Autodesk Inventor part; units mm, degrees
ref_plane "YZ Plane" through (0, 0, 0) normal (1, 0, 0) x (0, 1, 0)
ref_plane "XZ Plane" through (0, 0, 0) normal (0, 1, 0) x (-1, 0, 0)
ref_plane "XY Plane" through (0, 0, 0) normal (0, 0, 1) x (1, 0, 0)
sketch "Sketch1" plane through (0, 0, 0) normal (0, 0, 1) x (1, 0, 0)
  circle A0 centre (10, 20.7) radius 1.6
  line L0 (0, 0) -> (20.0001, 0)
  line L1 (0, 0) -> (0, 7)
  line L2 (20.0001, 0) -> (20.0001, 6.9998)
  line L3 (0, 7) -> (5.4723, 22.0351)
  line L4 (0, 7) -> (16, 7) construction
  line L5 (20.0001, 6.9998) -> (14.5277, 22.0349)
  line L6 (20.0001, 6.9998) -> (36.0001, 6.9998) construction
  arc A1 (14.5277, 22.0349) -> (5.4723, 22.0351) centre (10, 20.3869) ccw
  dimension "d17" = 7
  dimension "d18" = 6.9998
  dimension "d19" = 20.7
  dimension "d23" = 90
  dimension "d24" = 90
  dimension "d25" = 10
  dimension "d26" = 16
  dimension "d27" = 70
  dimension "d28" = 16
  dimension "d29" = 110
  dimension "d30" = 10
sketch "Sketch3" plane through (0, 0, 0) normal (0, 0, 1) x (1, 0, 0)
  point P0 (0, 0)
extrude "Extrusion1" add sketch "Sketch1" along normal blind 4.5
sketch "Sketch4" plane through (0, 0, 4.5) normal (0, 0, 1) x (1, 0, 0)
  line L0 (0, 7) -> (0, 0)
  line L1 (20.0001, 0) -> (20.0001, 6.9998)
  line L2 (0, 0) -> (20.0001, 0)
  line L3 (20.0001, 0) -> (20.0001, 6.9998)
  line L4 (3.884, 22.9404) -> (-0.0481, 7.0119)
  line L5 (20.0001, 6.9998) -> (0, 6.9998)
  line L6 (0, 7) -> (0, 0)
extrude "Extrusion2" add sketch "Sketch4" along normal blind 4.5
sketch "Sketch5" plane through (0, 0, 0) normal (0, -1, 0) x (1, 0, 0)
  circle A0 centre (5, 4) radius 0.5
  circle A1 centre (15, 4) radius 0.5
  line L0 (0, 0) -> (20.0001, 0)
  line L1 (0, 9) -> (20.0001, 9)
  dimension "d13" = 1
  dimension "d14" = 1
  dimension "d33" = 5
  dimension "d34" = 5
extrude "Extrusion3" cut sketch "Sketch5" against normal blind 5.5
properties part number "upper_deck_shaft_mount_for_AD"
Geometry: final body of the model. Coordinates: model frame, mm. A direction names the side the tool comes from. Coordinates: 2 decimals unless noted, no trailing zeros. Order: outer loops, then holes, each group sorted by start corner. A loop starts at its lowest first (then second) coordinate and runs counter-clockwise, first axis right, second up. Notation, with made-up numbers: M -28,41.5 L 21,41.5 A12 ccw 21,58.5 Z; hole C 75.25,75.25 d6. An arc over 180 degrees is marked long. Answer as CSV lines item,"result".
Q1. Section C-C on x = 9.25. Return the cut outline in (y, z), and give its area (3 significant figures).
Answers:
outline,"M 0,0 L 19.29,0 L 19.29,4.5 L 7,4.5 L 7,9 L 0,9 Z; M 22.11,0 L 25.15,0 L 25.15,4.5 L 22.11,4.5 Z"
area,"132 mm^2"
Q2. Section D-D on z = 4. Return the cut outline in (x, y).
Answers:
outline,"M 0,0 L 4.5,0 L 4.5,5.5 L 5.5,5.5 L 5.5,0 L 14.5,0 L 14.5,5.5 L 15.5,5.5 L 15.5,0 L 20,0 L 20,7 L 14.53,22.03 A4.82 ccw 5.47,22.04 L 0,7 Z; hole C 10,20.7 d3.2"
Q3. Line query: probe 1 along Z at (x, y) = (5, 2.45); probe 2 along Y at (x, z) = (10, 2.25); probe 3 along Z at (x, y) = (16, 8.75). Output: solid intervals per line, ascending. Write a range as [from, to].
Answers:
probe 1,"z = [0, 3.5], [4.5, 9]"
probe 2,"y = [0, 19.1], [22.3, 25.21]"
probe 3,"z = [0, 4.5]"
Q4. First-contact query: P1, Ø5, axis at x = 14, z = 7.5, coming from the +Y side; P2, Ø4, axis at y = 17.5, z = 4, coming from the -X side; P3, Ø1.5, axis at x = 7, y = 16.5, coming from the +Z side. Flat tips, straight axial feed; report the tip coordinate or a pass-through.
Answers:
P1,"stops at y = 7"
P2,"stops at x = 3.09"
P3,"stops at z = 4.5"
Q5. Set-up query: faces 5 (the cylindrical face through (8.73, 21.67, 2.22)), 6 (the cylindrical face through (14.935, 2.712, 4.496)), 7 (the flat face through (10, 14, 4.5)). Return all of +Z, -Z, +X, -X, +Y, -Y with unobstructed straight access to the full face (end or side cutting, diameter ignored); none if empty.
Answers:
face 5,"+Z, -Z"
face 6,"-Y"
face 7,"+Z, +X, -X, +Y"
Q6. Section B-B on y = 20.7. Return the cut outline in (x, z).
Answers:
outline,"M 4.99,0 L 8.4,0 L 8.4,4.5 L 4.99,4.5 Z; M 11.6,0 L 15.01,0 L 15.01,4.5 L 11.6,4.5 Z"
Q7. Section A-A on z = 1. Return the cut outline in (x, y).
Answers:
outline,"M 0,0 L 20,0 L 20,7 L 14.53,22.03 A4.82 ccw 5.47,22.04 L 0,7 Z; hole C 10,20.7 d3.2"
Q8. Draft query along X for faces 1 (the flat face through (20, 3, 4)), 2 (the cylindrical face through (9.918, 25.204, 2.218)), 3 (the flat face through (15, 5.5, 4)), 4 (the flat face through (10, 10, 0)). Return one class per face: pulls with the +X half, pulls with the -X half, needs draft (parallel to the pull), parting line crosses it, or undercut.
Answers:
face 1,"pulls with the +X half"
face 2,"parting line crosses it"
face 3,"undercut"
face 4,"needs draft"
